from build123d import *

# Parameters (mm, degrees)
F0_R     = 5
F1_DEPTH = 1.1
F0_R_2   = 10
F2_DEPTH = 0.6
F3_DEPTH = 0.6
F4_DEPTH = 1.1
F7_D     = 2.85
F7_DEPTH = 2.5
F7_TIP   = 0.8562263821


with BuildPart() as f1:
    # F0 (on Front) → F1 (new body)
    with BuildSketch(Plane.XZ):
        Circle(F0_R)
    extrude(amount=F1_DEPTH)

    # F0 (on Front) → F2 (join)
    with BuildSketch(Plane.XZ):
        Circle(F0_R_2)
        Circle(F0_R, mode=Mode.SUBTRACT)
    extrude(amount=F2_DEPTH)

    # F0 (on Front) → F3 (join)
    with BuildSketch(Plane.XZ):
        Circle(F0_R_2)
        Circle(F0_R, mode=Mode.SUBTRACT)
    extrude(amount=-F3_DEPTH)

    # F0 (on Front) → F4 (join)
    with BuildSketch(Plane.XZ):
        Circle(F0_R)
    extrude(amount=-F4_DEPTH)

    # F7
    with Locations(Plane(origin=(0, 1.1, 0), x_dir=(-1, 0, 0), z_dir=(0, 1, 0))):
        with Locations((0, 0)):
            Hole(F7_D / 2, depth=F7_DEPTH)
            with Locations((0, 0, -(F7_DEPTH + F7_TIP / 2))):  # 118° drill point
                Cone(0, F7_D / 2, F7_TIP, mode=Mode.SUBTRACT)


solid = f1.part
Work out the finished part from the listing and answer in its coordinate system (mm). A direction names the side the tool comes from. Give positions to 0.01 mm unless a question says otherwise; leave off trailing zeros. Write each loop counter-clockwise with the first axis right and the second up, starting at its lowest first coordinate (ties: lowest second). Pieces come first, ordered by that corner, then holes. Notation, with made-up numbers: (-12.75, 8) - (41.25, 8) arc R19 cw to (41.25, 32) - close; hole circle Ø3 at (-32, 48.25). An arc over 180 degrees is marked (long way). One line per item, written item: value. Start each with the question number.
1. For faces 4 (the flat face through (-5, 0.6, -2)), 5 (the cylindrical face through (-1.08, -0.85, -4.88)), 6 (the flat face through (-1.2, -1.1, 1.2)), determine the directions among +Z, -Z, +X, -X, +Y, -Y from which every point of the face is accessible in a straight line to the end or side of a thin tool.
2. Find section A-A (z = 0). Write down the section's boundary in (x, y) (3 decimals).
3. Find section D-D (z = -3). Write down the section's boundary in (x, y).
4. For a pull along X with two mould halves and no side action, classify faces 1 (the flat face through (-1.2, 1.1, 1.2)), 2 (the cylindrical face through (-2.17, -0.01, -9.76)), 3 (the cylindrical face through (-1.13, -0.02, -0.87)) as +X half, -X half, draft (parallel to the pull), parting line (faces both ways), or undercut.
5. Find section C-C (y = 0.15). Write down the section's boundary in (x, z) (3 decimals).
6. Given pin 1 (1.5 mm diameter, centred on x = -6, z = -0.5, fed in from -Y), flat-ended and moving along its own axis, determine where the tip first touches the part or whether it passes through.
7. Find section B-B (x = 0). Write down the section's boundary in (y, z) (3 decimals).
8. Consider probe 1 along Z at (x, y) = (0, 0.1) (3 decimals); probe 2 along Y at (x, z) = (1.75, 7); probe 3 along X at (y, z) = (0.65, 0.5). Determine where each line is inside the solid, lowest interval first.
Geometry results:
1. face 4: +Y
1. face 5: -Y
1. face 6: +Z, -Z, +X, -X, -Y
2. outline: (-10, -0.6) - (-5, -0.6) - (-5, -1.1) - (-1.425, -1.1) - (-1.425, 1.1) - (-5, 1.1) - (-5, 0.6) - (-10, 0.6) - close; (1.425, -1.1) - (5, -1.1) - (5, -0.6) - (10, -0.6) - (10, 0.6) - (5, 0.6) - (5, 1.1) - (1.425, 1.1) - close
3. outline: (-9.54, -0.6) - (-4, -0.6) - (-4, -1.1) - (4, -1.1) - (4, -0.6) - (9.54, -0.6) - (9.54, 0.6) - (4, 0.6) - (4, 1.1) - (-4, 1.1) - (-4, 0.6) - (-9.54, 0.6) - close
4. face 1: draft
4. face 2: parting line
4. face 3: undercut
5. outline: circle Ø20 at (0, 0); hole circle Ø2.85 at (0, 0)
6. pin 1: y = -0.6
7. outline: (-1.1, -5) - (-0.6, -5) - (-0.6, -10) - (0.6, -10) - (0.6, -5) - (1.1, -5) - (1.1, -1.425) - (-1.1, -1.425) - close; (-1.1, 1.425) - (1.1, 1.425) - (1.1, 5) - (0.6, 5) - (0.6, 10) - (-0.6, 10) - (-0.6, 5) - (-1.1, 5) - close
8. probe 1: -10 to -1.425, 1.425 to 10
8. probe 2: -0.6 to 0.6
8. probe 3: -4.97 to -1.33, 1.33 to 4.97
